from build123d import *

# Parameters (mm, degrees)
SKETCH1_R           = 4
BOSS_EXTRUDE1_DEPTH = 3
SKETCH2_W           = 30
SKETCH2_H           = 15
BOSS_EXTRUDE2_DEPTH = 4.5


with BuildPart() as part:
    # Sketch1 → Boss-Extrude1 (new body)
    with BuildSketch(Plane.XY):
        with BuildLine():
            Line((-21.706018243, 0), (-8.706018243, 0))
            Line((-8.706018243, 0), (-5, 5.3))
            Line((-5, 5.3), (5, 5.3))
            Line((5, 5.3), (8.706018243, 0))
            Line((8.706018243, 0), (21.706018243, 0))
            ThreePointArc((21.706018243, 0), (28.120289405, 7.841266738), (37.077384256, 3.108530697))
            Line((37.077384256, 3.108530697), (37.077384256, -8.994356464))
            Line((37.077384256, -8.994356464), (16, -18.2))
            Line((16, -18.2), (-16, -18.2))
            Line((-16, -18.2), (-37.077384256, -8.994356464))
            Line((-37.077384256, -8.994356464), (-37.077384256, 3.108530697))
            ThreePointArc((-37.077384256, 3.108530697), (-28.120289405, 7.841266738), (-21.706018243, 0))
        make_face()
        with Locations((-29.706018243, 0)):
            Circle(SKETCH1_R, mode=Mode.SUBTRACT)
        with Locations(Location((29.706018243, 0, 0), (0, 0, 180))):
            Circle(SKETCH1_R, mode=Mode.SUBTRACT)
    extrude(amount=BOSS_EXTRUDE1_DEPTH)

    # Sketch2 → Boss-Extrude2 (add)
    with BuildSketch(Plane.XY):
        with Locations((0, -9.7)):
            Rectangle(SKETCH2_W, SKETCH2_H)
    extrude(amount=-BOSS_EXTRUDE2_DEPTH)


solid = part.part
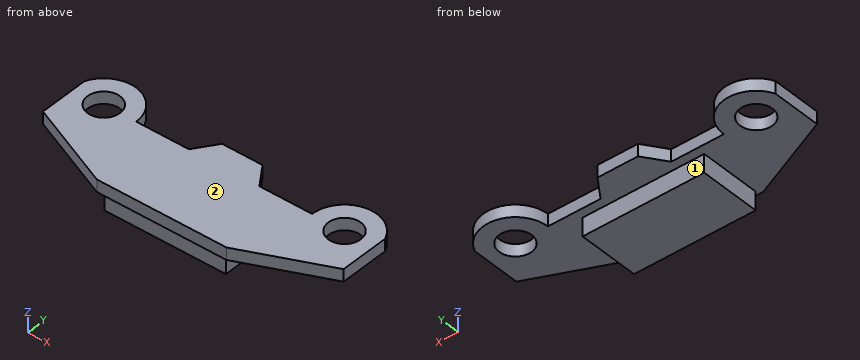
The listing builds one solid part. Answer for the finished solid, in the listing's coordinates (mm). Face numbers are marked on the shaded views. A direction names the side the tool comes from. Coordinates: 2 decimals unless noted, no trailing zeros. Loops run counter-clockwise (first coordinate to the right, second up) from the corner with the lowest first, then second, coordinate; pieces in that order, holes last. Notation, with made-up numbers: (20, -14.75) -> (75, -14.75) arc R9 cw to (75, 2.25) -> close; hole circle Ø10 at (33.25, -4). An arc over 180 degrees is marked (long way). Write item = value, one per line. Start each with the question number.
1) Given pin 1 Ø13 at (x, y) = (-29.71, 0) entering from -Z; pin 2 Ø1.5 at (x, z) = (-16.5, 1.5) entering from +Y; pin 3 Ø1.3 at (y, z) = (-6.5, -2) entering from -X; pin 4 Ø3.5 at (x, z) = (-5.5, -1.5) entering from -Y, each flat-ended and moving along its own axis, determine where each tip first touches the part or whether it passes through.
2) A cutting plane is placed at B-B (x = -26.5). Give the vertices of the cut face in (y, z).
3) Straight lines are drawn through the part: line 1 (X direction, y = -0.25, z = 0.5); line 2 (X direction, y = -5.25, z = -1.5); line 3 (Y direction, x = -2.5, z = -3.25). For each, find the intervals that lie inside material, in ascending order. Write a range as from..to.
4) A cutting plane is placed at A-A (y = -4.75). Give the vertices of the cut face in (x, z), then the cut area to 3 significant figures.
5) A cutting plane is placed at D-D (x = -13.5). Give the vertices of the cut face in (y, z), then the cut area to 3 significant figures.
6) A cutting plane is placed at C-C (z = -3.5). Give the vertices of the cut face in (x, y).
7) A tool of negligible diameter and unlimited length cuts with its end or side. For the marked faces 1 and 2, from which of +Z, -Z, +X, -X, +Y, -Y can it reach the whole face along a straight path? Write none if from no direction.
Responses:
q1.pin_1 = 0
q1.pin_2 = 0
q1.pin_3 = -15
q1.pin_4 = -18.2
q2.outline = (-13.61, 0) -> (-2.39, 0) -> (-2.39, 3) -> (-13.61, 3) -> close; (2.39, 0) -> (7.33, 0) -> (7.33, 3) -> (2.39, 3) -> close
q3.line_1 = -37.08..-33.7, -25.71..25.71, 33.7..37.08
q3.line_2 = -15..15
q3.line_3 = -17.2..-2.2
q4.outline = (-37.08, 0) -> (-15, 0) -> (-15, -4.5) -> (15, -4.5) -> (15, 0) -> (37.08, 0) -> (37.08, 3) -> (-37.08, 3) -> close
q4.area = 357 mm²
q5.outline = (-18.2, 0) -> (-17.2, 0) -> (-17.2, -4.5) -> (-2.2, -4.5) -> (-2.2, 0) -> (0, 0) -> (0, 3) -> (-18.2, 3) -> close
q5.area = 122 mm²
q6.outline = (-15, -17.2) -> (15, -17.2) -> (15, -2.2) -> (-15, -2.2) -> close
q7.face_1 = -Z, +X, -X, +Y
q7.face_2 = +Z, +X, -X, +Y, -Y
